```python
from build123d import *

# Parameters (mm, degrees)
SKETCH1_W             = 50
SKETCH1_H             = 45
BOSS_EXTRUDE1_DEPTH   = 6
SKETCH2_W             = 40
SKETCH2_H             = 35
SKETCH2_W_2           = 30
SKETCH2_H_2           = 26.25
CUT_EXTRUDE1_DEPTH    = 5
SKETCH8_W             = 27
SKETCH8_H             = 22
CUT_EXTRUDE2_DEPTH    = 3
SKETCH19_W            = 50
SKETCH19_H            = 45
SKETCH19_W_2          = 40
SKETCH19_H_2          = 35
CUT_EXTRUDE3_DEPTH    = 3
F_3_0MM_DOWEL_HOLE1_D = 3
F_3_0MM_DOWEL_HOLE2_D = 3


with BuildPart() as part:
    # Sketch1 → Boss-Extrude1 (new body)
    with BuildSketch(Plane.XY):
        Rectangle(SKETCH1_W, SKETCH1_H)
    extrude(amount=BOSS_EXTRUDE1_DEPTH)

    # Sketch2 → Cut-Extrude1 (cut)
    with BuildSketch(Plane(origin=(0, 0, 0), x_dir=(-1, 0, 0), z_dir=(0, 0, -1))):
        Rectangle(SKETCH2_W, SKETCH2_H)
        Rectangle(SKETCH2_W_2, SKETCH2_H_2, mode=Mode.SUBTRACT)
    extrude(amount=-CUT_EXTRUDE1_DEPTH, mode=Mode.SUBTRACT)

    # Sketch8 → Cut-Extrude2 (cut)
    with BuildSketch(Plane.XY.offset(6)):
        Rectangle(SKETCH8_W, SKETCH8_H)
    extrude(amount=-CUT_EXTRUDE2_DEPTH, mode=Mode.SUBTRACT)

    # Sketch19 → Cut-Extrude3 (cut)
    with BuildSketch(Plane(origin=(0, 0, 0), x_dir=(-1, 0, 0), z_dir=(0, 0, -1))):
        Rectangle(SKETCH19_W, SKETCH19_H)
        Rectangle(SKETCH19_W_2, SKETCH19_H_2, mode=Mode.SUBTRACT)
    extrude(amount=-CUT_EXTRUDE3_DEPTH, mode=Mode.SUBTRACT)

    # Ø3.0mm Dowel Hole1 (through all)
    with Locations(Plane(origin=(0, 0, 3), x_dir=(-1, 0, 0), z_dir=(0, 0, -1))):
        with Locations((-22.783121204, 14.123618146), (-22.783121204, -12.211210761), (-16.010997548, -20.358306406), (15.544462002, -20.358306406), (22.374348981, -12.211210761), (22.374348981, 14.123618146), (15.544462002, 19.971474687), (-16.010997548, 19.971474687)):
            Hole(F_3_0MM_DOWEL_HOLE1_D / 2)

    # Ø3.0mm Dowel Hole2 (through all)
    with Locations(Plane(origin=(0, 0, 0), x_dir=(-1, 0, 0), z_dir=(0, 0, -1))):
        with Locations((-11.409364772, 9.632100926), (-11.409364772, 4.733470352), (-11.409364772, 0), (-11.409364772, -4.688879244), (-11.409364772, -9.198386141), (-6.988624357, 7.056308434), (-6.988624357, 1.916488502), (-6.988624357, -2.81999563), (-6.988624357, -7.418696963), (-2.314259653, 9.632100926), (-2.314259653, 4.733470352), (2.260389176, 7.056308434), (6.385498081, 9.632100926), (6.385498081, 4.733470352), (10.808353766, 7.056308434), (-2.314259653, 0), (-2.314259653, -4.688879244), (-2.314259653, -9.198386141), (2.260389176, 1.916488502), (2.260389176, -2.81999563), (2.260389176, -7.418696963), (6.385498081, 0), (6.385498081, -4.688879244), (6.385498081, -9.198386141), (10.808353766, 1.916488502), (10.808353766, -2.81999563), (10.808353766, -7.418696963)):
            Hole(F_3_0MM_DOWEL_HOLE2_D / 2)


solid = part.part
```
CAD build for the part. Positions are in the model's coordinates, mm. A direction names the side the tool comes from. Round coordinates to 2 decimals unless told otherwise and drop trailing zeros. Write each loop counter-clockwise with the first axis right and the second up, starting at its lowest first coordinate (ties: lowest second). Pieces come first, ordered by that corner, then holes.
Item 1: Drop flat-ended pins along their axis: pin 1 Ø6.5 at (x, y) = (4.5, 0) entering from +Z; pin 2 Ø1.8 at (x, y) = (16.01, -20.36) entering from -Z; pin 3 Ø1.5 at (x, z) = (-15, 2) entering from -Y (3 decimals). Give the stop position or say it passes through.
Filled in:
pin 1: stops at z = 3
pin 2: passes through
pin 3: stops at y = -13.125
Item 2: Band-saw the part on C-C on y = 15. Write the cut outline in (x, z), then the cut area to 3 significant figures.
Filled in:
outline: (-25, 3) - (-23.59, 3) - (-23.59, 6) - (-25, 6) - close; (-21.16, 3) - (-20, 3) - (-20, 5) - (20, 5) - (20, 3) - (21.57, 3) - (21.57, 6) - (-21.16, 6) - close; (24, 3) - (25, 3) - (25, 6) - (24, 6) - close
area: 55.4 mm2
Item 3: Tool access for faces 1 (the cylindrical face through (-10.116, 5.726, 1.521)), 2 (the flat face through (13, 11, 5)), 3 (the flat face through (0, 17.5, 4)): list every direction of +Z, -Z, +X, -X, +Y, -Y with a clear straight run to the whole face (end or side of a thin tool).
Filled in:
face 1: +Z, -Z
face 2: +Z
face 3: -Z
Item 4: Band-saw the part on A-A on x = -16.5. Write the cut outline in (y, z), then the cut area to 3 significant figures.
Filled in:
outline: (-22.5, 3) - (-21.51, 3) - (-21.51, 6) - (-22.5, 6) - close; (-19.2, 3) - (-17.5, 3) - (-17.5, 5) - (17.5, 5) - (17.5, 3) - (18.82, 3) - (18.82, 6) - (-19.2, 6) - close; (21.13, 3) - (22.5, 3) - (22.5, 6) - (21.13, 6) - close
area: 51.1 mm2
Item 5: Drill centre lines: L1, parallel to X at y = 0.5, z = 3.4; L2, parallel to Y at x = 7, z = 2.8 (3 decimals); L3, parallel to Y at x = -11, z = 4 (3 decimals). Where is each one in solid material? Low to high.
Filled in:
L1: x = -25 to -20, -15 to -13.5, 13.5 to 15, 20 to 25
L2: y = -13.125 to -8.919, -5.919 to -4.32, -1.32 to 0.417, 3.416 to 5.556, 8.556 to 13.125
L3: y = -22.5 to -17.5, -13.125 to -11, 11 to 13.125, 17.5 to 22.5
Item 6: Band-saw the part on B-B on z = 1.2. Give the number of separate pieces and of enclosed holes in the cut face, then the cut area to 3 significant figures.
Filled in:
separate pieces: 1
enclosed holes: 27
area: 597 mm2
